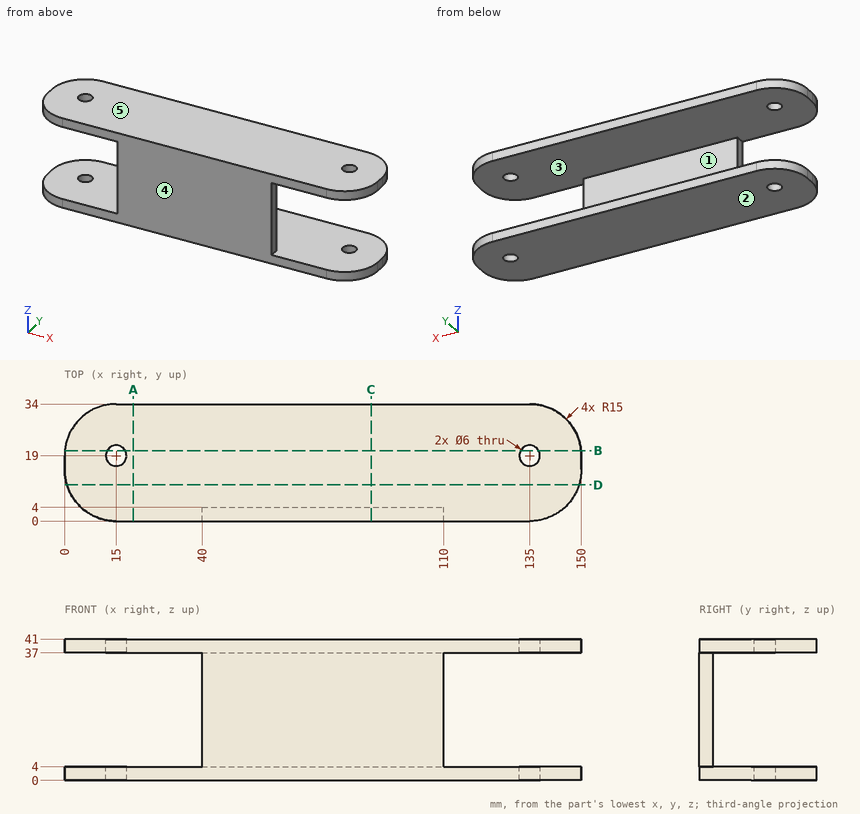
Here's the drawing with two shaded views (mm, measured from the low corner). I have some questions. A direction names the side the tool comes from. Give positions to 0.01 mm unless a question says otherwise; leave off trailing zeros. Write each loop counter-clockwise with the first axis right and the second up, starting at its lowest first coordinate (ties: lowest second). Pieces come first, ordered by that corner, then holes. Notation, with made-up numbers: (88, 70.5) -> (114, 70.5) arc R24 ccw to (114, 98.5) -> close; hole circle Ø7 at (-1.75, 20). An arc over 180 degrees is marked (long way). Use one line per item in the form item = value.
1) Suppose I cut it at C-C (x = 89). Please give me the cut outline in (y, z).
Verdict:
outline = (0, 0) -> (34, 0) -> (34, 4) -> (4, 4) -> (4, 37) -> (34, 37) -> (34, 41) -> (0, 41) -> close
2) On a 3-axis mill with a long thin cutter (end or side, diameter ignored), from which of +Z, -Z, +X, -X, +Y, -Y can I reach the whole of each face in a straight line? I mean the marked faces 1 and 2. Say none if no direction works.
Verdict:
face_1 = +X, -X, +Y
face_2 = -Z, +X, -X, +Y, -Y
3) Suppose I cut it at B-B (y = 20.5). Please give me the cut outline in (x, z).
Verdict:
outline = (0.08, 0) -> (12.4, 0) -> (12.4, 4) -> (0.08, 4) -> close; (0.08, 37) -> (12.4, 37) -> (12.4, 41) -> (0.08, 41) -> close; (17.6, 0) -> (132.4, 0) -> (132.4, 4) -> (17.6, 4) -> close; (17.6, 37) -> (132.4, 37) -> (132.4, 41) -> (17.6, 41) -> close; (137.6, 0) -> (149.92, 0) -> (149.92, 4) -> (137.6, 4) -> close; (137.6, 37) -> (149.92, 37) -> (149.92, 41) -> (137.6, 41) -> close
4) Suppose I cut it at A-A (x = 20). Please give me the cut outline in (y, z), and give its area (3 significant figures).
Verdict:
outline = (0, 0) -> (34, 0) -> (34, 4) -> (0, 4) -> close; (0, 37) -> (34, 37) -> (34, 41) -> (0, 41) -> close
area = 272 mm2
5) If I drill on L1, parallel to Z at x = 123.5, y = 26; L2, parallel to Y at x = 135, z = 38; L3, parallel to X at y = 3.5, z = 23.5, over which ranges is the centre line in solid material (lowest first)? Write a range as [from, to].
Verdict:
L1 = [0, 4], [37, 41]
L2 = [0, 16], [22, 34]
L3 = [40, 110]
6) I'm going to push flat-ended pins straight in: pin 1 (4.5 mm diameter, centred on y = 1, z = 18.5, fed in from +X); pin 2 (10 mm diameter, centred on x = 90, z = 25.5, fed in from +Y); pin 3 (1.2 mm diameter, centred on y = 1.5, z = 13.5, fed in from -X); pin 4 (5.5 mm diameter, centred on x = 135, y = 19, fed in from -Z). Where does each tip first touch, or does it pass through?
Verdict:
pin_1 = 110
pin_2 = 4
pin_3 = 40
pin_4 = through
7) Suppose I cut it at D-D (y = 10.5). Please give me the cut outline in (x, z).
Verdict:
outline = (0.69, 0) -> (149.31, 0) -> (149.31, 4) -> (0.69, 4) -> close; (0.69, 37) -> (149.31, 37) -> (149.31, 41) -> (0.69, 41) -> close
8) We'd pull the mould along Z, two halves only. Please class the marked faces 3, 4 and 5: +Z half, -Z half, draft (parallel to the pull), parting line (faces both ways), or undercut.
Verdict:
face_3 = undercut
face_4 = draft
face_5 = +Z half
